Autodesk Fusion 360 part; units mm, degrees
sketch "Sketch1" plane through (0, 0, 0) normal (0, 0, 1) x (1, 0, 0)
  line L0 (79.2263, -110) -> (-80.7737, -110)
  line L1 (-80.7737, -110) -> (-80.7737, 110)
  line L2 (-80.7737, 110) -> (79.2263, 110)
  line L3 (79.2263, 110) -> (79.2263, -110)
  line L4 (79.2263, -110) -> (-80.7737, 110) construction
  line L5 (-80.7737, -110) -> (79.2263, 110) construction
  point P0 (-0.7737, 0)
  dimension "d1" = 160
  dimension "d2" = 220
sketch "Sketch2" plane through (0, 0, 130) normal (0, 0, 1) x (-1, 0, 0)
  line L0 (-79.2263, -110) -> (80.7737, -110)
  line L1 (80.7737, -110) -> (80.7737, 110)
  line L2 (80.7737, 110) -> (-79.2263, 110)
  line L3 (-79.2263, 110) -> (-79.2263, -110)
  line L4 (-20, 110) -> (-79.2263, 29.9287)
sketch "Sketch3" plane through (0, 0, 0) normal (0, 0, 1) x (1, 0, 0)
  line L0 (85, -105) -> (-85, -105)
  line L1 (-85, -105) -> (-85, 105)
  line L2 (-85, 105) -> (85, 105)
  line L3 (85, 105) -> (85, -105)
  line L4 (85, -105) -> (-85, 105) construction
  line L5 (-85, -105) -> (85, 105) construction
  dimension "d7" = 170
  dimension "d8" = 210
extrude "Extrude3" add sketch "Sketch3" along normal blind 130
sketch "Sketch4" plane through (0, 0, 130) normal (0, 0, 1) x (-1, 0, 0)
  line L0 (-85, -105) -> (85, -105)
  line L1 (85, -105) -> (85, 105)
  line L2 (85, 105) -> (-85, 105)
  line L3 (-85, 105) -> (-85, -105)
  line L4 (-85, 105) -> (-15, 105)
  line L5 (-85, 101.8612) -> (-85, 31.8612)
  line L6 (-15, 105) -> (-85, 31.8612)
  line L7 (85, 105) -> (65, 105)
  line L8 (65, 105) -> (65, 65)
  line L9 (85, -105) -> (85, -65)
  line L10 (85, -65) -> (-65, -65)
  line L11 (-85, -105) -> (-85, -85)
  line L12 (-65, -65) -> (-85, -85)
  line L13 (85, -65) -> (5, -65)
  line L14 (5, -65) -> (5, -5)
  line L15 (5, -5) -> (65, 65)
  line L16 (85, -65) -> (45, -65)
  line L17 (45, -65) -> (45, -35)
  circle A0 centre (45, -35) radius 10
  dimension "d11" = 70
  dimension "d12" = 70
  dimension "d15" = 20
  dimension "d16" = 40
  dimension "d17" = 40
  dimension "d18" = 150
  dimension "d19" = 20
  dimension "d20" = 80
  dimension "d21" = 60
  dimension "d26" = 40
  dimension "d27" = 30
  dimension "d28" = 20
extrude "Extrude4" cut sketch "Sketch4" against normal blind 130 contours L2 L3 L4 L5 L6
extrude "Extrude5" cut sketch "Sketch4" against normal blind 60 contours L2 L3 L6 L8 L10 L12 L14 L15
extrude "Extrude6" cut sketch "Sketch4" against normal blind 20 contours A0 | L1 L2 L7 L8 L10 L13 L14 L15 L16
extrude "Extrude7" cut sketch "Sketch4" against normal blind 130 contours A0
sketch "Sketch5" plane through (0, 65, 0) normal (0, -1, 0) x (1, 0, 0)
  line L0 (65, 130) -> (-85, 130)
  line L1 (-85, 130) -> (-85, 110)
  line L2 (-85, 110) -> (-5, 110)
  line L3 (-5, 110) -> (-5, 70)
  line L4 (-5, 70) -> (65, 70)
  line L5 (65, 70) -> (65, 130)
  line L6 (65, 130) -> (35, 130)
  line L7 (35, 130) -> (35, 100)
  circle A0 centre (35, 100) radius 10
  dimension "d31" = 30
  dimension "d32" = 30
  dimension "d33" = 20
extrude "Extrude8" cut sketch "Sketch5" against normal blind 40 contours A0
sketch "Sketch6" plane through (85, 0, 0) normal (1, 0, 0) x (0, 1, 0)
  line L0 (85, 130) -> (85, 70)
  line L1 (85, 70) -> (-31.8612, 70)
  line L2 (-31.8612, 70) -> (-31.8612, 0)
  line L3 (-31.8612, 0) -> (105, 0)
  line L4 (105, 0) -> (105, 130)
  line L5 (105, 130) -> (85, 130)
  line L6 (105, 0) -> (105, 10)
  line L7 (105, 10) -> (-105.2237, 10)
  dimension "d36" = 10
extrude "Extrude9" cut sketch "Sketch6" against normal blind 300 contours L2 L3 L4 L6 L7
sketch "Sketch7" plane through (60.2783, -57.6914, 0) normal (0.7224, -0.6914, 0) x (0.6914, 0.7224, 0)
  line L0 (35.7542, 70) -> (-65.4846, 70)
  line L1 (-65.4846, 70) -> (-65.4846, 0)
  line L2 (-65.4846, 0) -> (35.7542, 0)
  line L3 (35.7542, 0) -> (35.7542, 10)
  line L4 (35.7542, 10) -> (35.7542, 70)
  line L5 (-65.4846, 0) -> (-65.4846, 10)
  line L6 (-65.4846, 10) -> (35.7542, 10)
  dimension "d39" = 10
extrude "Extrude10" cut sketch "Sketch7" against normal blind 399 contours L1 L2 L3 L5 L6
sketch "Sketch8" plane through (0, -105, 0) normal (0, -1, 0) x (1, 0, 0)
  line L0 (-65, 110) -> (-85, 110)
  line L1 (-85, 110) -> (-85, 0)
  line L2 (-85, 0) -> (15, 0)
  line L3 (15, 0) -> (15, 10)
  line L4 (15, 10) -> (15, 70)
  line L5 (15, 70) -> (-65, 70)
  line L6 (-65, 70) -> (-65, 110)
  line L7 (15, 10) -> (-85, 10)
extrude "Extrude11" cut sketch "Sketch8" against normal blind 300 contours L1 L2 L3 L7
Design review of the part built by this model. Coordinates are the model's own, in mm. A direction names the side the tool comes from. Give positions to 0.01 mm unless a question says otherwise; leave off trailing zeros. Loops run counter-clockwise (first coordinate to the right, second up) from the corner with the lowest first, then second, coordinate; pieces in that order, holes last. Notation, with made-up numbers: (-2.75, -1) -> (56.25, -1) arc R17 cw to (56.25, 12) -> close; hole circle Ø10 at (56, 84.25). An arc over 180 degrees is marked (long way). One line per question, with ' | ' between items. Start each with the question number.
(1) We need section D-D (z = 55). State the section outline as (x, y) points, and give its area (3 significant figures).
(2) Draft analysis for pull direction X (two halves, no side actions). For faces 4 (the face through (-1, 105, 69)), 5 (the face through (-85, -1, 69)), 6 (the face through (49.51, -68.94, 40.42)), 7 (the face through (-42.83, 44.76, 60.7)), state which applies: +X half, -X half, draft (parallel to the pull), parting line (faces both ways), or undercut.
(3) Insertion check: P1, Ø12, axis at y = 34.5, z = 97.5, coming from the +X side; P2, Ø18, axis at x = 35, z = 100, coming from the -Y side; P3, Ø10, axis at y = -57, z = 58, coming from the +X side; P4, Ø6, axis at x = 42.5, z = 102, coming from the -Y side. Each pin has a flat end and moves straight along its axis. Give the tip position at first contact, or say it passes through.
(4) For faces 1 (the face through (-65, -85, 90)), 2 (the face through (-53, -2, 110)), 3 (the face through (85, 38, 42)), list the 3-axis set-ups (+Z, -Z, +X, -X, +Y, -Y) from which the entire face can be reached by the end or side of a thin tool; tool diameter is ignored.
(5) We need section C-C (x = -51). State the section outline as (y, z) points.
(6) We need section A-A (z = 107.5). State the section outline as (x, y) points, and give its area (3 significant figures).
(7) For line 1 (Z direction, x = 35, y = 96); line 2 (X direction, y = 35, z = 82); line 3 (Y direction, x = 50, z = 112), list the stretches that pass through material, from the lowest coordinate up.
(8) We need section B-B (y = 35). State the section outline as (x, z) points, and give its area (3 significant figures).
The answers:
1) outline: (-85, -105) -> (15, -105) -> (85, -31.86) -> (85, 105) -> (-85, 105) -> close; hole circle Ø20 at (-45, 35) | area: 32,800 mm^2
2) face 4: draft | face 5: -X half | face 6: +X half | face 7: undercut
3) P1: stops at x = -5 | P2: passes through | P3: stops at x = 65.73 | P4: stops at y = 65
4) face 1: +Z, +X, -Y | face 2: +Z, +X, -X, -Y | face 3: +Z, -Z, +X, +Y, -Y
5) outline: (-105, 10) -> (27, 10) -> (27, 110) -> (-48.67, 110) -> (-48.67, 70) -> (-105, 70) -> close; (43, 10) -> (105, 10) -> (105, 130) -> (65, 130) -> (65, 110) -> (43, 110) -> close
6) outline: (-85, -105) -> (-65, -105) -> (-65, -65) -> (-5, 5) -> (-5, 65) -> (28.39, 65) -> (28.39, 105) -> (-85, 105) -> close; (41.61, 65) -> (65, 65) -> (85, 85) -> (85, 105) -> (41.61, 105) -> close; hole circle Ø20 at (-45, 35) | area: 14,900 mm^2
7) line 1: z = 10 to 90, 110 to 130 | line 2: x = -85 to -55, -35 to -5 | line 3: y = 65 to 105
8) outline: (-85, 10) -> (-55, 10) -> (-55, 110) -> (-85, 110) -> close; (-35, 10) -> (85, 10) -> (85, 70) -> (-5, 70) -> (-5, 110) -> (-35, 110) -> close | area: 11,400 mm^2
